Read the model definition and answer for the solid it produces. Units are mm, in the model's axes. A direction names the side the tool comes from. Round coordinates to 2 decimals unless told otherwise and drop trailing zeros. Write each loop counter-clockwise with the first axis right and the second up, starting at its lowest first coordinate (ties: lowest second). Pieces come first, ordered by that corner, then holes.
from build123d import *

# Parameters (mm, degrees)
F0_W     = 40
F0_H     = 40
F1_DEPTH = 40


with BuildPart() as f1:
    # F0 (on Front) → F1 (new body)
    with BuildSketch(Plane.XZ):
        with Locations((-40, 80)):
            Rectangle(F0_W, F0_H)
        with Locations((0, 80)):
            Rectangle(F0_W, F0_H)
        with Locations((40, 80)):
            Rectangle(F0_W, F0_H)
        with Locations((40, 40)):
            Rectangle(F0_W, F0_H)
        with Locations((40, 0)):
            Rectangle(F0_W, F0_H)
        Rectangle(F0_W, F0_H)
        with Locations((-40, 0)):
            Rectangle(F0_W, F0_H)
        with Locations((-40, -40)):
            Rectangle(F0_W, F0_H)
        with Locations((-40, -80)):
            Rectangle(F0_W, F0_H)
        with Locations((-40, 40)):
            Rectangle(F0_W, F0_H)
        Polygon((20, -60), (20, -20), (-20, -20), (0, -60), align=None)
        Polygon((40, -60), (20, -60), (20, -100), (60, -100), align=None)
        Polygon((20, -100), (20, -60), (0, -60), align=None)
        Polygon((40, -60), (20, -20), (20, -60), align=None)
    extrude(amount=F1_DEPTH)


solid = f1.part
Q1. Section C-C (y = -28) is taken. Determine the outline of the cut face in (x, z).
Verdict:
outline: (-60, -100) - (-20, -100) - (-20, -20) - (20, -100) - (60, -100) - (20, -20) - (60, -20) - (60, 100) - (-60, 100) - close; hole (-20, 20) - (20, 20) - (20, 60) - (-20, 60) - close
Q2. Determine the mould class of faces 4 (the flat face through (-20, -20, 40)), 5 (the flat face through (-40, -20, -100)), 6 (the flat face through (-20, -20, -61)) for opening direction Z: pulls with the +Z half, pulls with the -Z half, needs draft (parallel to the pull), parting line crosses it, or undercut.
Verdict:
face 4: undercut
face 5: pulls with the -Z half
face 6: needs draft
Q3. Straight lines are drawn through the part: probe 1 along X at (y, z) = (-15, 34.5); probe 2 along X at (y, z) = (-37.5, -23); probe 3 along Z at (x, y) = (2, -22.5). For each, find the intervals that lie inside material, in ascending order.
Verdict:
probe 1: x = -60 to -20, 20 to 60
probe 2: x = -60 to -20, -18.5 to 21.5
probe 3: z = -64 to 20, 60 to 100
Q4. Section B-B (z = 36) is taken. Determine the outline of the cut face in (x, y).
Verdict:
outline: (-60, -40) - (-20, -40) - (-20, 0) - (-60, 0) - close; (20, -40) - (60, -40) - (60, 0) - (20, 0) - close
Q5. Flat-ended cylindrical pins translate along their axes: pin 1 Ø3 at (x, z) = (17, 55.5) entering from -Y; pin 2 Ø10 at (x, y) = (2, -6) entering from -Z; pin 3 Ø20 at (y, z) = (-28, -53.5) entering from +X; pin 4 Ø4 at (y, z) = (-16, -63) entering from +X. Find the tip coordinate at first contact, or state that the pin passes through.
Verdict:
pin 1: passes through
pin 2: stops at z = -74
pin 3: stops at x = 41.75
pin 4: stops at x = 42.5
Q6. Which of the six approach directions +Z, -Z, +X, -X, +Y, -Y give full straight-line access (tool end or side, diameter ignored) to faces 1 (the flat face through (-0.3, -19.7, -59.4)), 2 (the flat face through (0, -20, 20)), 3 (the flat face through (40, -20, -20))?
Verdict:
face 1: -Z, +Y, -Y
face 2: +Y, -Y
face 3: +X, +Y, -Y
Q7. Section A-A (x = 52) is taken. Determine the outline of the cut face in (y, z), then the cut area to 3 significant figures.
Verdict:
outline: (-40, -100) - (0, -100) - (0, -84) - (-40, -84) - close; (-40, -20) - (0, -20) - (0, 100) - (-40, 100) - close
area: 5,440 mm2
